Build history of the part. All positions in model axes, mm. Face numbers are marked on the shaded views. Round coordinates to 2 decimals unless told otherwise and drop trailing zeros. Loops run counter-clockwise (first coordinate to the right, second up) from the corner with the lowest first, then second, coordinate; pieces in that order, holes last. Notation, with made-up numbers: (44.5, 39) - (92.5, 39) arc R27 ccw to (92.5, 71) - close; hole circle Ø2 at (22.25, 60.5). An arc over 180 degrees is marked (long way). Answer as CSV lines item,"result". Start each with the question number.
Autodesk Inventor part; units mm, degrees
ref_plane "YZ Plane" through (0, 0, 0) normal (1, 0, 0) x (0, 1, 0)
ref_plane "XZ Plane" through (0, 0, 0) normal (0, 1, 0) x (-1, 0, 0)
ref_plane "XY Plane" through (0, 0, 0) normal (0, 0, 1) x (1, 0, 0)
sketch "Sketch1" plane through (0, 0, 0) normal (0, 0, 1) x (1, 0, 0)
  line L0 (0, 0) -> (0, 5.08)
  line L1 (0, 5.08) -> (1.8, 5.08)
  line L2 (1.8, 5.08) -> (1.8, 6.35)
  line L3 (1.8, 6.35) -> (5.95, 6.35)
  line L4 (5.95, 6.35) -> (5.95, 12.85)
  line L5 (5.95, 12.85) -> (6.05, 12.85)
  line L6 (6.05, 12.85) -> (6.05, 4.85)
  line L7 (6.05, 4.85) -> (6.55, 4.85)
  line L8 (6.55, 4.85) -> (6.55, 0)
  line L9 (0, 0) -> (11.8727, 0) construction
  line L10 (0, 0) -> (6.55, 0)
  dimension "d0" = 5.08
  dimension "d1" = 1.8
  dimension "d2" = 1.27
  dimension "d3" = 4.15
  dimension "d4" = 6.5
  dimension "d5" = 0.1
  dimension "d6" = 8
  dimension "d7" = 0.5
revolve "Revolution1" add sketch "Sketch1" angle 360 about axis through (0, 0, 0) along (1, 0, 0)
sketch "Sketch2" plane through (6.55, 0, 0) normal (1, 0, 0) x (0, 0, -1)
  circle A0 centre (0, 0) radius 4
  dimension "d9" = 8
extrude "Extrusion1" cut sketch "Sketch2" against normal blind 10
sketch "Sketch3" plane through (1.8, 0, 0) normal (-1, 0, 0) x (0, 0, 1)
  circle A0 centre (0, 0) radius 6.35
  point P0 (0, -6.35)
ref_plane "Work Plane1" through (1.8, -6.35, 0) normal (0, -1, 0) x (1, 0, 0)
sketch "Sketch4" plane through (1.8, -6.35, 0) normal (0, -1, 0) x (1, 0, 0)
  circle A0 centre (2.125, 0) radius 1.5
  line L0 (4.25, -12.85) -> (4.25, 12.85)
  line L1 (0, -6.35) -> (0, 6.35)
  point P0 (-1.8, 0)
  dimension "d12" = 3
  dimension "d14" = 4.25
  dimension "d15" = 2.125
hole "Hole1" at (3.925, -6.35, 0) direction (0, 1, 0) diameter 1.6942 depth 6.637 tip angle 118
equation "\"d15\" = 0.5 * d14"
properties part number "Tarcza impulsowa HEDS-5140"
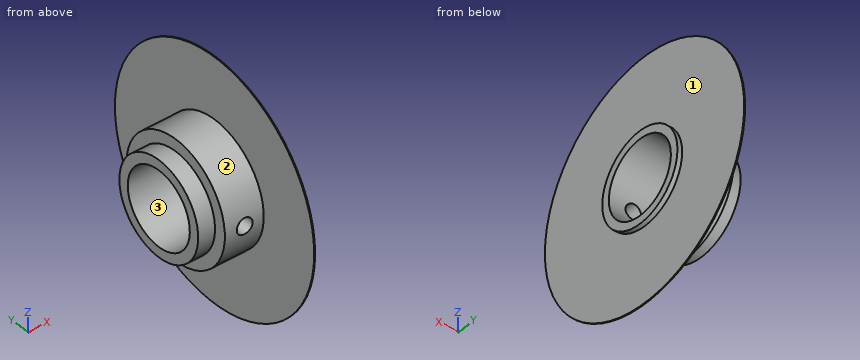
Q1. Band-saw the part on B-B, the plane y = 0. List the corners of the cut face in (x, z), then the cut area to 3 significant figures.
Q2. Pin check, flat tips, straight feed: pin 1 Ø1.5 at (x, z) = (3.925, 0) entering from -Y; pin 2 Ø5 at (y, z) = (9.5, -2.5) entering from -X; pin 3 Ø6 at (y, z) = (-6.5, 4.5) entering from +X. Stop position of each tip, or through.
Q3. Band-saw the part on D-D, the plane x = 0.5. List the corners of the cut face in (y, z), then the cut area to 3 significant figures.
Q4. Band-saw the part on C-C, the plane z = 3.5. List the corners of the cut face in (x, y).
Q5. Band-saw the part on A-A, the plane z = 0. List the corners of the cut face in (x, y), then the cut area to 3 significant figures.
Q6. Two-plate mould, pull along Z, no slides. Class the marked faces 1, 2 and 3: released by +Z, released by -Z, zero draft, split by the parting line, or undercut.
Q7. Wall check: probe 1 along X at (y, z) = (-4.5, 0); probe 2 along Y at (x, z) = (0.5, -3.5); probe 3 along Z at (x, y) = (3, -1.5). Give the ranges that are in metal, low to high. Write a range as [from, to].
Reported:
1,outline,"(0, -5.08) - (1.8, -5.08) - (1.8, -6.35) - (5.95, -6.35) - (5.95, -12.85) - (6.05, -12.85) - (6.05, -4.85) - (6.55, -4.85) - (6.55, -4) - (0, -4) - close; (0, 4) - (6.55, 4) - (6.55, 4.85) - (6.05, 4.85) - (6.05, 12.85) - (5.95, 12.85) - (5.95, 6.35) - (1.8, 6.35) - (1.8, 5.08) - (0, 5.08) - close"
1,area,"26.0 mm2"
2,pin 1,"stops at y = 3.93"
2,pin 2,"stops at x = 5.95"
2,pin 3,"stops at x = 6.05"
3,outline,"circle Ø10.16 at (0, 0); hole circle Ø8 at (0, 0)"
3,area,"30.8 mm2"
4,outline,"(0, -3.68) - (1.8, -3.68) - (1.8, -5.3) - (5.95, -5.3) - (5.95, -12.36) - (6.05, -12.36) - (6.05, -3.36) - (6.55, -3.36) - (6.55, -1.94) - (0, -1.94) - close; (0, 1.94) - (6.55, 1.94) - (6.55, 3.36) - (6.05, 3.36) - (6.05, 12.36) - (5.95, 12.36) - (5.95, 5.3) - (1.8, 5.3) - (1.8, 3.68) - (0, 3.68) - close"
5,outline,"(0, -5.08) - (1.8, -5.08) - (1.8, -6.35) - (3.08, -6.35) - (3.08, -4) - (0, -4) - close; (0, 4) - (6.55, 4) - (6.55, 4.85) - (6.05, 4.85) - (6.05, 12.85) - (5.95, 12.85) - (5.95, 6.35) - (1.8, 6.35) - (1.8, 5.08) - (0, 5.08) - close; (4.77, -6.35) - (5.95, -6.35) - (5.95, -12.85) - (6.05, -12.85) - (6.05, -4.85) - (6.55, -4.85) - (6.55, -4) - (4.77, -4) - close"
5,area,"22.0 mm2"
6,face 1,"zero draft"
6,face 2,"split by the parting line"
6,face 3,"undercut"
7,probe 1,"x = [0, 3.08], [4.77, 6.55]"
7,probe 2,"y = [-3.68, -1.94], [1.94, 3.68]"
7,probe 3,"z = [-6.17, -3.71], [3.71, 6.17]"
